Autodesk Inventor part; units mm, degrees
ref_plane "YZ Plane" through (0, 0, 0) normal (1, 0, 0) x (0, 1, 0)
ref_plane "XZ Plane" through (0, 0, 0) normal (0, 1, 0) x (-1, 0, 0)
ref_plane "XY Plane" through (0, 0, 0) normal (0, 0, 1) x (1, 0, 0)
sketch "草圖1" plane through (0, 0, 0) normal (0, 1, 0) x (-1, 0, 0)
  arc A0 (1.8, 0) -> (-1.8, 0) centre (0, 0) ccw
  line L0 (0, 0) -> (0, -20) construction
  arc A1 (-1.8, -20) -> (1.8, -20) centre (0, -20) ccw
  arc A2 (3.5, 0) -> (-3.5, 0) centre (0, 0) ccw
  line L1 (1.8, 0) -> (1.8, -20)
  line L2 (-1.8, 0) -> (-1.8, -20)
  line L3 (0, -20) -> (0, -35) construction
  line L4 (3.5, 0) -> (3.5, -31.8)
  line L5 (-3.5, 0) -> (-3.5, -31.8)
  circle A3 centre (0, -35) radius 1.25
  line L6 (0, -35) -> (0, -25.4) construction
  line L7 (0, -35) -> (0, -31.8) construction
  line L8 (0, -31.8) -> (0, -28.6) construction
  line L9 (0, -28.6) -> (0, -25.4) construction
  circle A4 centre (0, -31.8) radius 1.25
  circle A5 centre (0, -28.6) radius 1.25
  circle A6 centre (0, -25.4) radius 1.25
  line L10 (3.5, -31.8) -> (2.1243, -35.7414)
  line L11 (-3.5, -31.8) -> (-2.1243, -35.7414)
  arc A7 (-2.1243, -35.7414) -> (2.1243, -35.7414) centre (0, -35) ccw
  dimension "d0" = 3.6
  dimension "d1" = 20
  dimension "d2" = 3.6
  dimension "d3" = 7
  dimension "d5" = 15
  dimension "d9" = 2.5
  dimension "d13" = 3.2
  dimension "d14" = 3.2
  dimension "d15" = 3.2
  dimension "d16" = 2.5
  dimension "d17" = 2.5
  dimension "d18" = 2.5
extrude "Extrusion3" add sketch "草圖1" along normal blind 3
properties part number "轉向軸"
Could you check a few things on this model? Use its own coordinates, in mm. A direction names the side the tool comes from. Round coordinates to 2 decimals unless told otherwise and drop trailing zeros. Write each loop counter-clockwise with the first axis right and the second up, starting at its lowest first coordinate (ties: lowest second). Pieces come first, ordered by that corner, then holes. Notation, with made-up numbers: (16.5, 11) -> (58.5, 11) arc R18 ccw to (58.5, 23) -> close; hole circle Ø8 at (73.5, 18.5). An arc over 180 degrees is marked (long way). Use a Markdown table: item, result.
1. Please list where these lines run through material, in increasing order: probe 1 along Z at (x, y) = (0, 2.3); probe 2 along X at (y, z) = (1.35, -4); probe 3 along Z at (x, y) = (1, 1.95).
Answer key:
| item | result |
|---|---|
| probe 1 | z = -37.25 to -36.25, -33.75 to -33.05, -30.55 to -29.85, -27.35 to -26.65, -24.15 to -21.8, 1.8 to 3.5 |
| probe 2 | x = -3.5 to -1.8, 1.8 to 3.5 |
| probe 3 | z = -37.02 to -35.75, -34.25 to -32.55, -31.05 to -29.35, -27.85 to -26.15, -24.65 to -21.5, 1.5 to 3.35 |
2. If we section it at A-A (z = -28.6): List the corners of the cut face in (x, y) for me.
Answer key:
| item | result |
|---|---|
| outline | (-3.5, 0) -> (-1.25, 0) -> (-1.25, 3) -> (-3.5, 3) -> close; (1.25, 0) -> (3.5, 0) -> (3.5, 3) -> (1.25, 3) -> close |
3. Which directions (+Z, -Z, +X, -X, +Y, -Y) give clear straight access to the entire face, cutting with the end or side of a thin tool? Please do faces 4 (the face through (0.1, 1.5, 3.5)), 5 (the face through (0, 1.5, -21.8)).
Answer key:
| item | result |
|---|---|
| face 4 | +Z, +Y, -Y |
| face 5 | +Y, -Y |
4. If we section it at B-B (y = 2.6): List the corners of the cut face in (x, z) for me.
Answer key:
| item | result |
|---|---|
| outline | (-3.5, -31.8) -> (-2.12, -35.74) arc R2.25 ccw to (2.12, -35.74) -> (3.5, -31.8) -> (3.5, 0) arc R3.5 ccw to (-3.5, 0) -> close; hole (-1.8, -20) arc R1.8 ccw to (1.8, -20) -> (1.8, 0) arc R1.8 ccw to (-1.8, 0) -> close; hole circle Ø2.5 at (0, -35); hole circle Ø2.5 at (0, -31.8); hole circle Ø2.5 at (0, -28.6); hole circle Ø2.5 at (0, -25.4) |
5. For pin 1 Ø1 at (x, y) = (2, 2) entering from +Z; pin 2 Ø1.5 at (x, z) = (0, -35) entering from -Y; pin 3 Ø1.5 at (x, y) = (1, 2) entering from +Z, each with a flat end and sliding along its axis, tell me the tip position at first contact or that it passes through.
Answer key:
| item | result |
|---|---|
| pin 1 | stops at z = 3.16 |
| pin 2 | passes through |
| pin 3 | stops at z = 3.49 |
6. If we section it at D-D (z = -18): List the corners of the cut face in (x, y) for me, then the cut area to 3 significant figures.
Answer key:
| item | result |
|---|---|
| outline | (-3.5, 0) -> (-1.8, 0) -> (-1.8, 3) -> (-3.5, 3) -> close; (1.8, 0) -> (3.5, 0) -> (3.5, 3) -> (1.8, 3) -> close |
| area | 10.2 mm^2 |
7. If we section it at C-C (x = 0): List the corners of the cut face in (y, z) for me.
Answer key:
| item | result |
|---|---|
| outline | (0, -37.25) -> (3, -37.25) -> (3, -36.25) -> (0, -36.25) -> close; (0, -33.75) -> (3, -33.75) -> (3, -33.05) -> (0, -33.05) -> close; (0, -30.55) -> (3, -30.55) -> (3, -29.85) -> (0, -29.85) -> close; (0, -27.35) -> (3, -27.35) -> (3, -26.65) -> (0, -26.65) -> close; (0, -24.15) -> (3, -24.15) -> (3, -21.8) -> (0, -21.8) -> close; (0, 1.8) -> (3, 1.8) -> (3, 3.5) -> (0, 3.5) -> close |
8. We'd pull the mould along Z, two halves only. Please class faces 1 (the face through (2.822, 1.479, -33.743)), 2 (the face through (0.27, 1.48, -33.78)), 3 (the face through (-2, 0, -17)): +Z half, -Z half, draft (parallel to the pull), parting line (faces both ways), or undercut.
Answer key:
| item | result |
|---|---|
| face 1 | -Z half |
| face 2 | undercut |
| face 3 | draft |
